```python
from build123d import *

# Parameters (mm, degrees)
F0_R      = 38.1
F0_R_2    = 34.29
F1_DEPTH  = 20.32
F4_R      = 38.1
F3_R      = 12.7
F6_T      = -2.54
F5_FACE_R = 34.29
F7_DEPTH  = 3.556
F7_TAPER  = 8
F9_R      = 40.932761629
F10_DEPTH = 3
F11_R     = 35.392761629
F12_DEPTH = 4.6


# Not quite as in the source:
# - a fillet or chamfer that OpenCascade refuses, or shapes differently, is made with other operations: its cross-section is extruded or revolved along the edge and cut away or added


with BuildPart() as f1:
    # F0 (on Top) → F1 (new body)
    with BuildSketch(Plane.XY):
        Circle(F0_R)
        Circle(F0_R_2, mode=Mode.SUBTRACT)
    extrude(amount=F1_DEPTH)

    # F4 (on face) → F5 section 0
    with BuildSketch(Plane.XY.offset(20.32)):
        Circle(F4_R)
    # F3 (on offset) → F5 section 1
    with BuildSketch(Plane.XY.offset(71.12)):
        Circle(F3_R)
    loft()

    # F6
    f6_openings = [f1.faces().sort_by_distance(p)[0] for p in [
        (0, 0, 71.12),
    ]]
    offset(amount=F6_T, openings=f6_openings, kind=Kind.INTERSECTION)

    # F5_face (on face) → F7 (cut)
    with BuildSketch(Plane(origin=(0, 0, 20.32), x_dir=(1, 0, 0), z_dir=(0, 0, -1))):
        Circle(F5_FACE_R)
    extrude(amount=-F7_DEPTH, taper=F7_TAPER, mode=Mode.SUBTRACT)

    # F8: fillet of radius 14.4671225158 on 1 edges, made by hand

    # F8_s1 → F8_t2 (revolve, cut)
    with BuildSketch(Plane.XZ):
        with BuildLine():
            ThreePointArc((15.7937700832, 64.9324598335), (13.2958276301, 68.4758321875), (9.8601936686, 71.12))
            Line((9.8601936686, 71.12), (12.7, 71.12))
            Line((12.7, 71.12), (15.7937700832, 64.9324598335))
        make_face()
    revolve(axis=Axis((0, 0, 71.12), (0, 0, 1)), mode=Mode.SUBTRACT)

    # F9 (on Top) → F10 (join)
    with BuildSketch(Plane.XY):
        Circle(F9_R)
    extrude(amount=-F10_DEPTH)

    # F11 (on face) → F12 (cut)
    with BuildSketch(Plane(origin=(0, 0, -3), x_dir=(1, 0, 0), z_dir=(0, 0, -1))):
        Circle(F11_R)
    extrude(amount=-F12_DEPTH, mode=Mode.SUBTRACT)


solid = f1.part
```
Source: CAD feature listing. Evaluate the final solid. Frame: model axes, mm. A direction names the side the tool comes from. Coordinates: 2 decimals unless noted, no trailing zeros. Order: outer loops, then holes, each group sorted by start corner. A loop starts at its lowest first (then second) coordinate and runs counter-clockwise, first axis right, second up. Notation, with made-up numbers: M 44,58.5 L 84,58.5 A25 ccw 84,88.5 Z; hole C -18,0 d10. An arc over 180 degrees is marked long. Write each question's results on one line, items separated by ' | '. Start each with the question number.
1) Draft query along Y for faces 4 (the face through (-18, 31, -3)), 5 (the face through (-30.235, -23.183, 10.018)), 6 (the face through (18.3, -28.6, 22.7)). Return one class per face: released by +Y, released by -Y, zero draft, split by the parting line, or undercut.
2) Section query B-B (z = 54). Return the cut outline in (x, y).
3) Line query: line 1 (Y direction, x = 0, z = -0.9); line 2 (Y direction, x = 0, z = 5.75); line 3 (Z direction, x = -21.5, y = 34). Output: solid intervals per line, ascending. Write a range as from..to.
4) Section query A-A (z = 9). Return the cut outline in (x, y).
5) Contact query for flat-ended pins moving along their axis: pin 1 Ø8 at (x, z) = (18, 26) entering from +Y; pin 2 Ø12 at (x, z) = (-22.5, 4.5) entering from +Y; pin 3 Ø5 at (y, z) = (-1.5, 34) entering from +X. Output: stop coordinate, or through.
6) Access query for faces 1 (the face through (22.01, 34.51, -1.48)), 2 (the face through (27.1, -27.1, 0)), 3 (the face through (-19, -29, 1.6)). Directions: +Z, -Z, +X, -X, +Y, -Y. A direction counts if a zero-diameter tool reaches every point of the face in a straight line with its end or side. Return the directions, or none.
Answers:
1) face 4: zero draft | face 5: split by the parting line | face 6: undercut
2) outline: C 0,0 d42.52; hole C 0,0 d36.84
3) line 1: y = -40.93..-35.39, 35.39..40.93 | line 2: y = -38.1..-34.29, 34.29..38.1 | line 3: z = -3..0
4) outline: C 0,0 d76.2; hole C 0,0 d68.58
5) pin 1: stops at y = 33.4 | pin 2: stops at y = 36.5 | pin 3: stops at x = 32.48
6) face 1: +Z, -Z | face 2: +Z | face 3: -Z
